from build123d import *

# Parameters (mm, degrees)
SKIZZE1_R                            = 2.5
SKIZZE1_R_2                          = 5
SKIZZE1_R_3                          = 3.25
SKIZZE1_R_4                          = 4
AUFSATZ_LINEAR_AUSTRAGEN2_DEPTH      = 1.5
AUFSATZ_LINEAR_AUSTRAGEN2_DEPTH_BACK = 0.0001


with BuildPart() as part:
    # Skizze1 → Aufsatz-Linear austragen2 (new body, two sides)
    with BuildSketch(Plane.XY) as aufsatz_linear_austragen2_sk:
        Polygon((-241.005153528, -55), (-216.005153528, -55), (-221.628929887, -79.35925162), (62.246314842, -114.231101944), (68.994846472, -85), (68.994846472, -70), (48.994846472, -70), (48.994846472, 70), (68.994846472, 70), (68.994846472, 85), (62.246314842, 114.231101944), (-221.628929887, 79.35925162), (-216.005153528, 55), (-241.005153528, 55), (-246.005153528, 20), (-246.005153528, -20), align=None)
        with Locations((-228.505153528, -47.5)):
            Circle(SKIZZE1_R, mode=Mode.SUBTRACT)
        with Locations((-228.505153528, -32.5)):
            Circle(SKIZZE1_R, mode=Mode.SUBTRACT)
        with Locations((-228.505153528, -21.5)):
            Circle(SKIZZE1_R, mode=Mode.SUBTRACT)
        with Locations((-225.505153528, -27)):
            Circle(SKIZZE1_R, mode=Mode.SUBTRACT)
        with Locations((-228.505153528, 47.5)):
            Circle(SKIZZE1_R, mode=Mode.SUBTRACT)
        with Locations((8.994846472, 40)):
            Circle(SKIZZE1_R_2, mode=Mode.SUBTRACT)
        with Locations((-201.005153528, -32.5)):
            Circle(SKIZZE1_R_3, mode=Mode.SUBTRACT)
        with Locations((-181.005153528, 0)):
            Circle(SKIZZE1_R_3, mode=Mode.SUBTRACT)
        with Locations((-81.005153528, -32.5)):
            Circle(SKIZZE1_R_2, mode=Mode.SUBTRACT)
        with Locations((8.994846472, -40)):
            Circle(SKIZZE1_R_2, mode=Mode.SUBTRACT)
        with Locations((-201.005153528, 32.5)):
            Circle(SKIZZE1_R_3, mode=Mode.SUBTRACT)
        with Locations((-81.005153528, 32.5)):
            Circle(SKIZZE1_R_2, mode=Mode.SUBTRACT)
        with Locations((-188.77946315, -70.434923444)):
            Circle(SKIZZE1_R_4, mode=Mode.SUBTRACT)
        with Locations((-188.77946315, 70.434923444)):
            Circle(SKIZZE1_R_4, mode=Mode.SUBTRACT)
    extrude(amount=AUFSATZ_LINEAR_AUSTRAGEN2_DEPTH)
    extrude(aufsatz_linear_austragen2_sk.sketch, amount=-AUFSATZ_LINEAR_AUSTRAGEN2_DEPTH_BACK)


solid = part.part
Model file for the job. Use its own axes, mm. Give positions to 0.01 mm unless a question says otherwise; leave off trailing zeros. Order: outer loops, then holes, each group sorted by start corner. A loop starts at its lowest first (then second) coordinate and runs counter-clockwise, first axis right, second up. Notation, with made-up numbers: (-7, 21) - (35, 21) arc R23 ccw to (35, 55) - close; hole circle Ø4 at (9, -18.75). An arc over 180 degrees is marked (long way). One line per item, written item: value.
Item 1: Slice it at B-B (z = 0.65). Give the number of separate pieces and of enclosed holes in the cut face, then the cut area to 3 significant figures.
Response values:
separate pieces: 1
enclosed holes: 14
area: 55,300 mm2
Item 2: Slice it at D-D (x = -138.5). List the corners of the cut face in (y, z).
Response values:
outline: (-89.57, 0) - (89.57, 0) - (89.57, 1.5) - (-89.57, 1.5) - close
Item 3: Pin check, flat tip, straight feed: pin 1 Ø0.5 at (x, z) = (-232, 1) entering from -Y. Stop position of the tip, or through.
Response values:
pin 1: y = -55
Item 4: Wall check: line 1 (Y direction, x = -79, z = 1.25); line 2 (X direction, y = -30.5, z = 0.6); line 3 (X direction, y = -9, z = 0.35). Give the ranges that are in metal, low to high.
Response values:
line 1: -96.88 to -37.08, -27.92 to 27.92, 37.08 to 96.88
line 2: -244.51 to -230.01, -227.01 to -203.57, -198.44 to -85.59, -76.42 to 48.99
line 3: -246.01 to 48.99
Item 5: Slice it at C-C (x = -104). List the corners of the cut face in (y, z), then the cut area to 3 significant figures.
Response values:
outline: (-93.81, 0) - (93.81, 0) - (93.81, 1.5) - (-93.81, 1.5) - close
area: 281 mm2
Item 6: Two-plate mould, pull along X, no slides. Class faces 1 (the flat face through (-91, 2, 1.5)), 2 (the flat face through (65.573, -99.82, 0.76)), 3 (the cylindrical face through (-184.252, 0.143, 0.739)): released by +X, released by -X, zero draft, split by the parting line, or undercut.
Response values:
face 1: zero draft
face 2: released by +X
face 3: undercut
Item 7: Slice it at A-A (y = 0). List the corners of the cut face in (x, z).
Response values:
outline: (-246.01, 0) - (-184.26, 0) - (-184.26, 1.5) - (-246.01, 1.5) - close; (-177.76, 0) - (48.99, 0) - (48.99, 1.5) - (-177.76, 1.5) - close
